from build123d import *

# Parameters (mm, degrees)
F0_R     = 16.845
F0_R_2   = 9.75
F1_DEPTH = 28.21
F0_R_3   = 4.825
F2_DEPTH = 28.21


with BuildPart() as f1:
    # F0 (on Top) → F1 (new body)
    with BuildSketch(Plane.XY):
        Circle(F0_R)
        Circle(F0_R_2, mode=Mode.SUBTRACT)
    extrude(amount=F1_DEPTH)

    # F0 (on Top) → F2 (join)
    with BuildSketch(Plane.XY):
        Circle(F0_R_2)
        Circle(F0_R_3, mode=Mode.SUBTRACT)
    extrude(amount=F2_DEPTH)

    # F3 (on Front) → F4 (revolve, cut)
    with BuildSketch(Plane.XZ):
        with BuildLine():
            Line((15.345, 15.3), (16.845, 15.3))
            Line((16.845, 15.3), (16.845, 19.3))
            Line((16.845, 19.3), (15.345, 19.3))
            ThreePointArc((15.345, 19.3), (13.345, 17.3), (15.345, 15.3))
        make_face()
    revolve(axis=Axis((0, 0, 14.105), (0, 0, 1)), mode=Mode.SUBTRACT)

    # F5 (on Front) → F6 (revolve, cut)
    with BuildSketch(Plane.XZ):
        with BuildLine():
            ThreePointArc((5.680042, 19.3), (5.794747, 19.869563), (6.068315, 20.382124))
            Line((6.068315, 20.382124), (9.75, 28.21))
            Line((9.75, 28.21), (0, 28.21))
            Line((0, 28.21), (0, 19.3))
            Line((0, 19.3), (5.680042, 19.3))
        make_face()
        with BuildLine():
            ThreePointArc((5.721742, 18.774543), (5.683505, 19.035892), (5.680042, 19.3))
            Line((5.680042, 19.3), (0, 19.3))
            Line((0, 19.3), (0, 0))
            Line((0, 0), (9.75, 0))
            Line((9.75, 0), (5.721742, 18.774543))
        make_face()
    revolve(axis=Axis((0, 0, 14.105), (0, 0, 1)), mode=Mode.SUBTRACT)


solid = f1.part
Source: CAD feature listing. Evaluate the final solid. Frame: model axes, mm. Coordinates: 2 decimals unless noted, no trailing zeros. Loops run counter-clockwise (first coordinate to the right, second up) from the corner with the lowest first, then second, coordinate; pieces in that order, holes last. Notation, with made-up numbers: (70.25, 61) - (119.25, 61) arc R23 cw to (119.25, 100) - close; hole circle Ø1 at (23, 41). An arc over 180 degrees is marked (long way). One line per question, with ' | ' between items.
1) Pull-direction query (Z, two-part tool) for faces 1 (the face through (15, 4, 19.3)), 2 (the face through (7.3, -7.3, 28.21)), 3 (the face through (-15, 4, 15.3)), 4 (the face through (-2.2, 16.7, 7.5)); classes: released by +Z, released by -Z, zero draft, split by the parting line, or undercut.
Report:
face 1: undercut | face 2: released by +Z | face 3: undercut | face 4: zero draft
2) Line query: line 1 along Z through (x, y) = (-15, 4); line 2 along X through (y, z) = (3, 4.5); line 3 along X through (y, z) = (-4.5, 8.75). Output: solid intervals per line, ascending.
Report:
line 1: z = 0 to 15.3, 19.3 to 28.21 | line 2: x = -16.58 to -8.26, 8.26 to 16.58 | line 3: x = -16.23 to -6.46, 6.46 to 16.23
3) Section D-D, the plane z = 12.75. Return loops of the section in (x, y) (3 decimals), then the cut area to 3 significant figures.
Report:
outline: circle Ø33.69 at (0, 0); hole circle Ø14.029 at (0, 0) | area: 737 mm²
4) Section C-C, the plane z = 5.5. Return loops of the section in (x, y) (3 decimals), then the cut area to 3 significant figures.
Report:
outline: circle Ø33.69 at (0, 0); hole circle Ø17.14 at (0, 0) | area: 661 mm²
5) First-contact query: P1, Ø6, axis at y = 11.5, z = 22.5, coming from the -X side; P2, Ø3, axis at x = -4.5, y = -6, coming from the +Z side; P3, Ø2, axis at x = -12.5, z = 18.5, coming from the +Y side. Flat tips, straight axial feed; report the tip coordinate or a pass-through.
Report:
P1: stops at x = -14.54 | P2: stops at z = 26.62 | P3: stops at y = 11.92
6) Section A-A, the plane x = 0. Return loops of the section in (y, z) (3 decimals), then the cut area to 3 significant figures.
Report:
outline: (-16.845, 0) - (-9.75, 0) - (-5.722, 18.775) arc R2 ccw to (-5.68, 19.3) arc R2 ccw to (-6.068, 20.382) - (-9.75, 28.21) - (-16.845, 28.21) - (-16.845, 19.3) - (-15.345, 19.3) arc R2 cw to (-15.345, 15.3) - (-16.845, 15.3) - close; (5.68, 19.3) arc R2 ccw to (5.722, 18.775) - (9.75, 0) - (16.845, 0) - (16.845, 15.3) - (15.345, 15.3) arc R2 cw to (15.345, 19.3) - (16.845, 19.3) - (16.845, 28.21) - (9.75, 28.21) - (6.068, 20.382) arc R2 ccw to start | area: 493 mm²
